```python
from build123d import *

# Parameters (mm, degrees)
F0_R     = 25
F1_DEPTH = 48
F2_W     = 66.378064
F2_H     = 62.903502
F3_DEPTH = 56
F4_W     = 78.902334
F4_H     = 58.748622
F5_DEPTH = 61.5
F6_R     = 15
F7_DEPTH = 105.3


with BuildPart() as f1:
    # F0 (on Front) → F1 (new body)
    with BuildSketch(Plane.XZ):
        Circle(F0_R)
    extrude(amount=-F1_DEPTH)

    # F2 (on Front) → F3 (join)
    with BuildSketch(Plane.XZ):
        Rectangle(F2_W, F2_H)
    extrude(amount=F3_DEPTH)

    # F4 (on Top) → F5 (join, symmetric)
    with BuildSketch(Plane.XY):
        Rectangle(F4_W, F4_H)
    extrude(amount=F5_DEPTH, both=True)

    # F6 (on face) → F7 (cut)
    with BuildSketch(Plane(origin=(0, 48, 0), x_dir=(-1, 0, 0), z_dir=(0, 1, 0))):
        Circle(F6_R)
    extrude(amount=-F7_DEPTH, mode=Mode.SUBTRACT)


solid = f1.part
```
Geometry: final body of the model. Coordinates: model frame, mm. A direction names the side the tool comes from. Give positions to 0.01 mm unless a question says otherwise; leave off trailing zeros. Order: outer loops, then holes, each group sorted by start corner. A loop starts at its lowest first (then second) coordinate and runs counter-clockwise, first axis right, second up. Notation, with made-up numbers: M 84,23 L 143,23 A19 ccw 143,27 Z; hole C 0,67 d4. An arc over 180 degrees is marked long. Answer as CSV lines item,"result". Start each with the question number.
1) Mould query, pull axis X, two halves, no side actions, for faces 5 (the flat face through (11, 48, -11)), 6 (the cylindrical face through (14.985, -3.272, 0.66)), 7 (the flat face through (-33.189, -43, 0)). Classes: +X half, -X half, draft (parallel to the pull), parting line (faces both ways), or undercut.
2) First-contact query: P1, Ø10, axis at y = 34.5, z = -26, coming from the +X side; P2, Ø13.5, axis at y = -49, z = -4.5, coming from the -X side; P3, Ø8, axis at x = -5.5, y = -36.5, coming from the +Z side. Flat tips, straight axial feed; report the tip coordinate or a pass-through.
3) Cut plane B-B (x = 0). Output: boundary loops of the cut face in (y, z), then the cut area to 3 significant figures.
4) Line query: line 1 (Z direction, x = 0, y = 11); line 2 (Y direction, x = 24.5, z = -27.5); line 3 (Y direction, x = 29, z = 32). Output: solid intervals per line, ascending. Write a range as from..to.
5) Cut plane D-D (y = 38.5). Output: boundary loops of the cut face in (x, z), then the cut area to 3 significant figures.
6) Cut plane C-C (x = -31). Output: boundary loops of the cut face in (y, z), then the cut area to 3 significant figures.
7) Set-up query: faces 1 (the flat face through (0, -43, -31.452)), 2 (the flat face through (0, -43, 31.452)), 3 (the flat face through (33.189, -43, 0)), 4 (the cylindrical face through (23.846, 38.557, 7.509)). Return all of +Z, -Z, +X, -X, +Y, -Y with unobstructed straight access to the full face (end or side cutting, diameter ignored); none if empty.
8) Cut plane A-A (z = 0). Output: boundary loops of the cut face in (x, y).
Findings below:
1,face 5,"draft"
1,face 6,"undercut"
1,face 7,"-X half"
2,P1,"stops at x = 13.56"
2,P2,"stops at x = -33.19"
2,P3,"stops at z = 31.45"
3,outline,"M -56,-31.45 L -29.37,-31.45 L -29.37,-61.5 L 29.37,-61.5 L 29.37,-25 L 48,-25 L 48,-15 L -56,-15 Z; M -56,15 L 48,15 L 48,25 L 29.37,25 L 29.37,61.5 L -29.37,61.5 L -29.37,31.45 L -56,31.45 Z"
3,area,"6,710 mm²"
4,line 1,"z = -61.5..-15, 15..61.5"
4,line 2,"y = -56..29.37"
4,line 3,"y = -29.37..29.37"
5,outline,"C 0,0 d50; hole C 0,0 d30"
5,area,"1,260 mm²"
6,outline,"M -56,-31.45 L -29.37,-31.45 L -29.37,-61.5 L 29.37,-61.5 L 29.37,61.5 L -29.37,61.5 L -29.37,31.45 L -56,31.45 Z"
6,area,"8,900 mm²"
7,face 1,"-Z, +X, -X, -Y"
7,face 2,"+Z, +X, -X, -Y"
7,face 3,"+Z, -Z, +X, -Y"
7,face 4,"+Y"
8,outline,"M -39.45,-29.37 L -33.19,-29.37 L -33.19,-56 L -15,-56 L -15,48 L -25,48 L -25,29.37 L -39.45,29.37 Z; M 15,-56 L 33.19,-56 L 33.19,-29.37 L 39.45,-29.37 L 39.45,29.37 L 25,29.37 L 25,48 L 15,48 Z"
